CAD build for the part. Positions are in the model's coordinates, mm. A direction names the side the tool comes from. Give positions to 0.01 mm unless a question says otherwise; leave off trailing zeros. Write each loop counter-clockwise with the first axis right and the second up, starting at its lowest first coordinate (ties: lowest second). Pieces come first, ordered by that corner, then holes. Notation, with made-up numbers: (1, -1.75) -> (36, -1.75) arc R29 cw to (36, 26.25) -> close; hole circle Ø11 at (34, 11). An arc over 180 degrees is marked (long way). Use one line per item in the form item = value. Start each with the question number.
from build123d import *

# Parameters (mm, degrees)
ESQUISSE1_W             = 304
ESQUISSE1_H             = 48
BOSS_EXTRU_1_DEPTH      = 24
ESQUISSE2_R             = 4.5
ENL_V_MAT_EXTRU_1_DEPTH = 156.743378671
ESQUISSE3_R             = 7
ENL_V_MAT_EXTRU_2_DEPTH = 12


with BuildPart() as part:
    # Esquisse1 → Boss.-Extru.1 (new body)
    with BuildSketch(Plane(origin=(0, 0, 0), x_dir=(1, 0, 0), z_dir=(0, 1, 0))):
        Rectangle(ESQUISSE1_W, ESQUISSE1_H)
    extrude(amount=BOSS_EXTRU_1_DEPTH)

    # Esquisse2 → Enlèv. mat.-Extru.1 (cut, through all)
    with BuildSketch(Plane(origin=(0, 24, 0), x_dir=(1, 0, 0), z_dir=(0, 1, 0))):
        with Locations(Location((0, 0, 0), (0, 0, 270))):
            Circle(ESQUISSE2_R)
    extrude(amount=-ENL_V_MAT_EXTRU_1_DEPTH, mode=Mode.SUBTRACT)

    # Esquisse3 → Enlèv. mat.-Extru.2 (cut)
    with BuildSketch(Plane.XZ):
        with Locations(Location((0, 0, 0), (0, 0, 270))):
            Circle(ESQUISSE3_R)
    extrude(amount=-ENL_V_MAT_EXTRU_2_DEPTH, mode=Mode.SUBTRACT)


solid = part.part
1) Cut at A-A (z = 0). Give the cut face in (x, y).
2) Wall check: line 1 along X through (y, z) = (9.25, 0); line 2 along X through (y, z) = (15.5, 0). Give the ranges that are in metal, low to high. Write a range as from..to.
3) Pin check, flat tips, straight feed: pin 1 (8.5 mm diameter, centred on x = 0, z = 0, fed in from +Y); pin 2 (10.5 mm diameter, centred on x = 0, z = 0, fed in from -Y). Stop position of each tip, or through.
4) 3-axis set-ups, long thin cutter, end or side, ignore diameter. For faces 4 (the face through (-5, 12, 0)), 5 (the face through (-2, 12, 24)): which of +Z, -Z, +X, -X, +Y, -Y reach the whole face in a straight line?
5) Two-plate mould, pull along X, no slides. Class faces 1 (the face through (-2, 24, -6)), 2 (the face through (-6.834, 5.916, 1.517)), 3 (the face through (-152, 12, 0)): released by +X, released by -X, zero draft, split by the parting line, or undercut.
Final values:
q1.outline = (-152, 0) -> (-7, 0) -> (-7, 12) -> (-4.5, 12) -> (-4.5, 24) -> (-152, 24) -> close; (4.5, 12) -> (7, 12) -> (7, 0) -> (152, 0) -> (152, 24) -> (4.5, 24) -> close
q2.line_1 = -152..-7, 7..152
q2.line_2 = -152..-4.5, 4.5..152
q3.pin_1 = through
q3.pin_2 = 12
q4.face_4 = -Y
q4.face_5 = +Z, +X, -X, +Y, -Y
q5.face_1 = zero draft
q5.face_2 = undercut
q5.face_3 = released by -X
